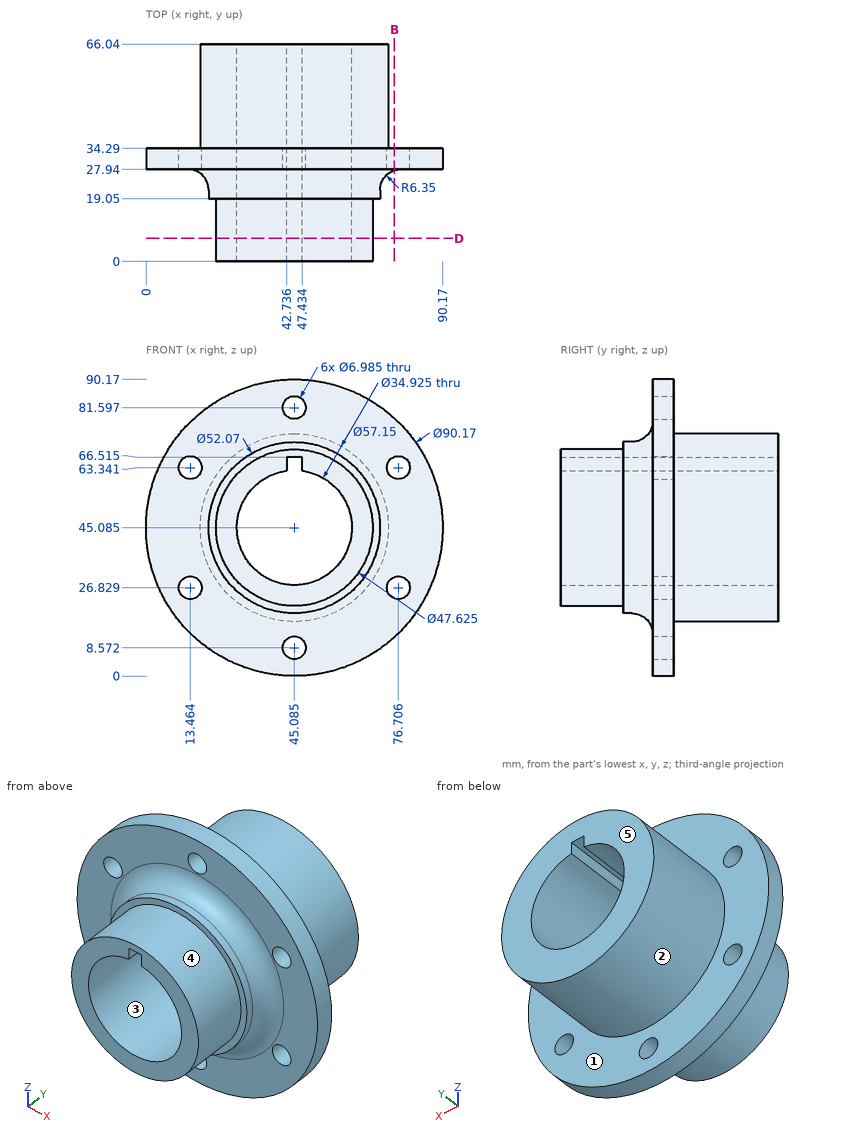
The drawing under review shows one solid part. Ordinate dimensions are in mm from its lowest x, y, z. A direction names the side the tool comes from. Give positions to 0.01 mm unless a question says otherwise; leave off trailing zeros. Order: outer loops, then holes, each group sorted by start corner. A loop starts at its lowest first (then second) coordinate and runs counter-clockwise, first axis right, second up. Notation, with made-up numbers: (36, 12.25) -> (87, 12.25) arc R37 cw to (87, 51.25) -> close; hole circle Ø5 at (48.25, 80.25). An arc over 180 degrees is marked (long way). Write item = value, one per line. Start each with the question number.
(1) We need section B-B on x = 75.5. State how many separate pieces and enclosed holes the cut face has, plus the area to 3 significant figures.
(2) For the marked faces 4 and 5, list the 3-axis set-ups (+Z, -Z, +X, -X, +Y, -Y) from which the entire face can be reached by the end or side of a thin tool; tool diameter is ignored.
(3) We need section D-D on y = 7. Write out the cut boundary in (x, z) (1 decimal).
(4) To check wall thickness, follow line 1 along Z through (x, y) = (44.5, 13.5) (1 decimal); line 2 along Y through (x, z) = (20, 22); line 3 along Z through (x, y) = (32.5, 30) (1 decimal). State the ranges of each line that lie inside material, in increasing order.
(5) Mouldability with a two-part tool opening along X and no side actions: class the marked faces 1, 2 and 3 as +X half, -X half, draft (parallel to the pull), parting line (faces both ways), or undercut.
(6) For pin 1 (1.2 mm diameter, centred on y = 38, z = 64, fed in from -X); pin 2 (6.5 mm diameter, centred on x = 76.71, z = 26.83, fed in from -Y); pin 3 (5 mm diameter, centred on x = 38, y = 41, fed in from +Z); pin 4 (4 mm diameter, centred on x = 47, y = 18, fed in from +Z), all flat-tipped, find the tip position at first contact; note any pin that passes through.
Numbers:
q1.separate_pieces = 3
q1.enclosed_holes = 0
q1.area = 343 mm^2
q2.face_4 = -Y
q2.face_5 = +Z, -Z, +X, -X, +Y
q3.outline = circle Ø47.6 at (45.1, 45.1); hole (42.7, 62.4) arc R17.5 ccw (long way) to (47.4, 62.4) -> (47.4, 66.5) -> (42.7, 66.5) -> close
q4.line_1 = 21.3 to 27.6, 66.5 to 68.9
q4.line_2 = 27.94 to 34.29
q4.line_3 = 1.8 to 33, 57.2 to 88.4
q5.face_1 = draft
q5.face_2 = parting line
q5.face_3 = undercut
q6.pin_1 = 23.15
q6.pin_2 = through
q6.pin_3 = 73.29
q6.pin_4 = 71.12
